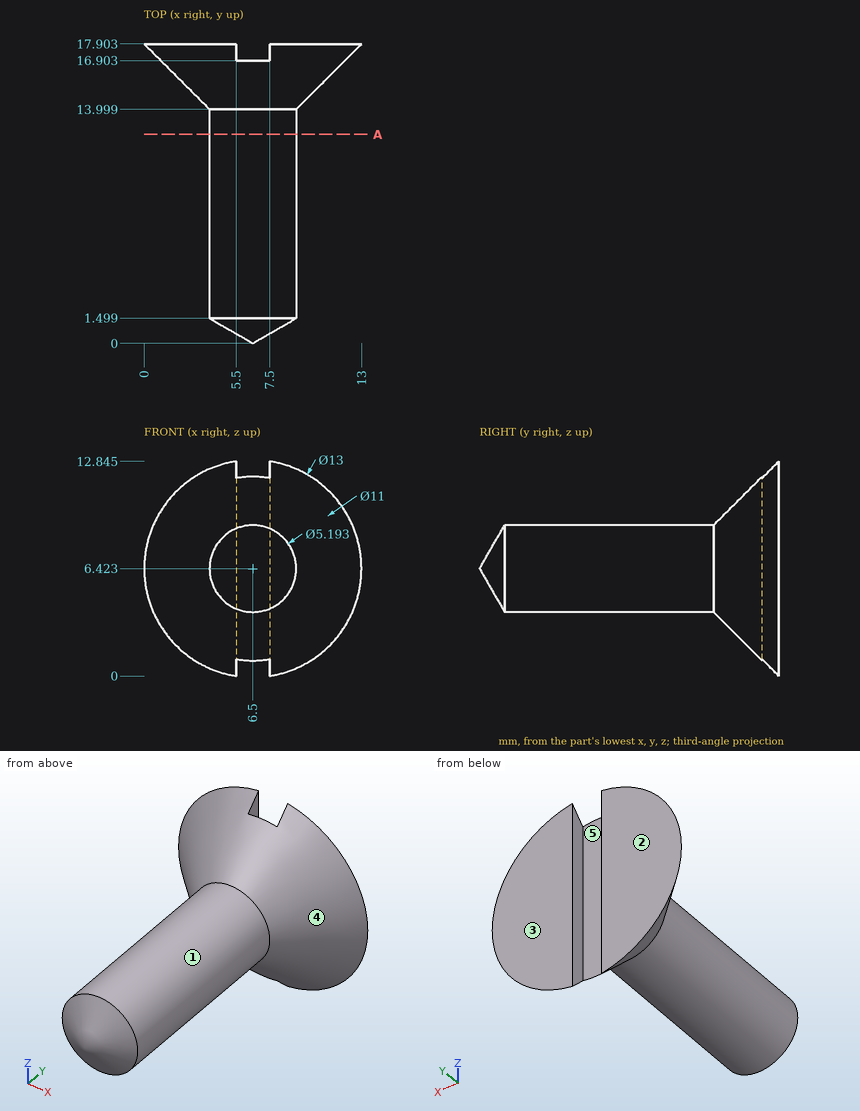
Geometry check sheet. Reference: drawing and pictorial views, mm from the part's lowest x, y, z. A direction names the side the tool comes from. Round coordinates to 2 decimals unless told otherwise and drop trailing zeros. Loops run counter-clockwise (first coordinate to the right, second up) from the corner with the lowest first, then second, coordinate; pieces in that order, holes last. Notation, with made-up numbers: (73, -36) - (90, -36) arc R26 cw to (90, 3) - close; hole circle Ø6 at (81.5, 86.25). An arc over 180 degrees is marked (long way). Use a Markdown table: item, result.
Q1. Cross-section at A-A on y = 12.5. Record the cut outline in (x, z).
Solutions:
| item | result |
|---|---|
| outline | circle Ø5.19 at (6.5, 6.42) |
Q2. Go/stop test with flat-tipped pins: P1, Ø4, axis at x = 9, y = 4, coming from the +Z side; P2, Ø1.1, axis at y = 17.5, z = 4.5, coming from the +X side; P3, Ø6, axis at y = 2, z = 5, coming from the -X side; P4, Ø2, axis at x = 11, y = 7, coming from the +Z side. Record where each tip stops, or that it passes through.
Solutions:
| item | result |
|---|---|
| P1 | stops at z = 8.97 |
| P2 | stops at x = 12.81 |
| P3 | stops at x = 3.9 |
| P4 | passes through |
Q3. Draft check along X on the marked faces 3, 4 and 5. Enter one of: released by +X, released by -X, zero draft, split by the parting line, or undercut.
Solutions:
| item | result |
|---|---|
| face 3 | zero draft |
| face 4 | split by the parting line |
| face 5 | undercut |
Q4. Access from +Z, -Z, +X, -X, +Y, -Y to the whole of each face (thin tool, end or side, straight path). Record for the marked faces 1 and 2.
Solutions:
| item | result |
|---|---|
| face 1 | -Y |
| face 2 | +Z, -Z, +X, -X, +Y |
Q5. Material ranges on line 1 (Z direction, x = 6.5, y = 5.75); line 2 (Y direction, x = 6.5, z = 9.25); line 3 (Y direction, x = 5, z = 7), recorded low to high.
Solutions:
| item | result |
|---|---|
| line 1 | z = 3.83 to 9.02 |
| line 2 | y = 14.23 to 16.9 |
| line 3 | y = 0.93 to 17.9 |
